Check sheet for the modelled part. Datum: model origin and axes. Units: mm. Face numbers are marked on the shaded views. A direction names the side the tool comes from. Give positions to 0.01 mm unless a question says otherwise; leave off trailing zeros. Loops run counter-clockwise (first coordinate to the right, second up) from the corner with the lowest first, then second, coordinate; pieces in that order, holes last. Notation, with made-up numbers: M -40,-18 L -5,-18 A12 ccw -5,-7 Z; hole C 87.25,13 d7. An arc over 180 degrees is marked long. Put each result on its own line as item: value. Start each with the question number.
```python
from build123d import *

# Parameters (mm, degrees)
F0_R     = 7.5
F1_DEPTH = 2
F2_R     = 3
F3_DEPTH = 22
F5_D     = 5
F6_R     = 4
F6_R_2   = 3
F7_DEPTH = 2.5
F8_SIZE  = 0.2


with BuildPart() as f1:
    # F0 (on Top) → F1 (new body)
    with BuildSketch(Plane.XY):
        Circle(F0_R)
    extrude(amount=F1_DEPTH)

    # F2 (on face) → F3 (join)
    with BuildSketch(Plane.XY.offset(2)):
        Circle(F2_R)
    extrude(amount=F3_DEPTH)

    # F5 (through all)
    with Locations(Plane(origin=(0, 0, 0), x_dir=(1, 0, 0), z_dir=(0, 0, -1))):
        with Locations((0, 0)):
            Hole(F5_D / 2)

    # F6 (on face) → F7 (join)
    with BuildSketch(Plane.XY.offset(2)):
        Circle(F6_R)
        Circle(F6_R_2, mode=Mode.SUBTRACT)
    extrude(amount=F7_DEPTH)

    # F8
    f8_edges = [f1.edges().sort_by_distance(p)[0] for p in [
        (-3, 0, 24),
        (-7.5, 0, 2),
        (-7.5, 0, 0),
        (-3, 0, 4.5),
        (-4, 0, 4.5),
        (-4, 0, 2),
        (-2.5, 0, 0),
        (-2.5, 0, 24),
    ]]
    chamfer(f8_edges, length=F8_SIZE)


solid = f1.part
```
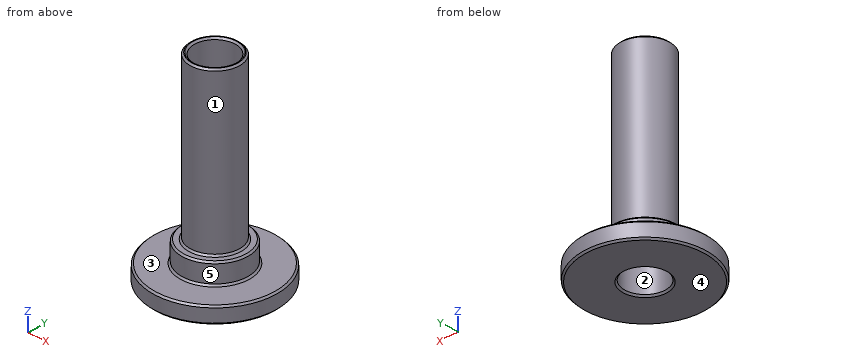
Q1. Access from +Z, -Z, +X, -X, +Y, -Y to the whole of each face (thin tool, end or side, straight path). Record for the marked faces 4 and 5.
Q2. Depth check by flat-ended pin: P1, Ø8, axis at y = 4.5, z = 13.5, coming from the +X side; P2, Ø1, axis at x = -0.5, z = 17, coming from the -Y side. Enter the tip coordinate at first touch or a pass-through.
Q3. Section check C-C, the plane z = 11. Record the cut outline in (x, y), then the cut area to 3 significant figures.
Q4. Thickness scan on line 1 along Y through (x, z) = (0, 19); line 2 along Z through (x, y) = (5.25, -1); line 3 along X through (y, z) = (-2, 9). Record the ranges inside material, lowest first. Write a range as [from, to].
Q5. Section check D-D, the plane z = 3.5. Record the cut outline in (x, y).
Q6. Mould release check, pull along Y, two halves, no side actions. Record for the marked faces 1, 2 and 3: pulls with the +Y half, pulls with the -Y half, needs draft (parallel to the pull), parting line crosses it, or undercut.
Found:
1. face 4: -Z, +X, -X, +Y, -Y
1. face 5: +Z
2. P1: stops at x = 2.96
2. P2: stops at y = -3
3. outline: C 0,0 d6; hole C 0,0 d5
3. area: 8.64 mm^2
4. line 1: y = [-3, -2.5], [2.5, 3]
4. line 2: z = [0, 2]
4. line 3: x = [-2.24, -1.5], [1.5, 2.24]
5. outline: C 0,0 d8; hole C 0,0 d5
6. face 1: parting line crosses it
6. face 2: undercut
6. face 3: needs draft
